For this review, take the finished solid that the model builds, in its own axes (mm). Coordinates: 2 decimals unless noted, no trailing zeros. Write each loop counter-clockwise with the first axis right and the second up, starting at its lowest first coordinate (ties: lowest second). Pieces come first, ordered by that corner, then holes. Notation, with made-up numbers: (79.25, 82.25) -> (118.25, 82.25) arc R12 cw to (118.25, 94.25) -> close; hole circle Ø3 at (29.5, 40.5). An arc over 180 degrees is marked (long way). Put each result on its own line as item: value. Start each with the question number.
Item 1: To check wall thickness, follow L1, parallel to X at y = -27, z = 11; L2, parallel to Z at x = 126, y = -24. State the ranges of each line that lie inside material, in increasing order.
Item 2: Consider section B-B on y = -17.5. Give the boundary of the cut face in (x, z).
Item 3: Insertion check: P1, Ø5, axis at y = -27.5, z = 28, coming from the +X side; P2, Ø5, axis at y = -51, z = 34.5, coming from the +X side; P3, Ø1, axis at y = -68, z = 18, coming from the +X side. Each pin has a flat end and moves straight along its axis. Give the tip position at first contact, or say it passes through.
Item 4: Consider section A-A on z = 40. Give the boundary of the cut face in (x, y).
Item 5: The part is to be moulded in two halves that separate along Y. For faces 1 (the flat face through (62, 0, 22)), 2 (the cylindrical face through (130.739, -27.575, 22.656)), 3 (the cylindrical face through (133.556, -60.157, 23.441)), 4 (the flat face through (138.43, -27, 27)), say which applies: +Y half, -Y half, draft (parallel to the pull), parting line (faces both ways), or undercut.
```python
from build123d import *

# Parameters (mm, degrees)
F0_W     = 125.73
F0_H     = 43.18
F1_DEPTH = 80.518
F2_R     = 6.35
F3_DEPTH = 19.05
F2_R_2   = 4.7625
F4_DEPTH = 12.7
F5_R     = 3.175
F6_R     = 2.54


with BuildPart() as f1:
    # F0 (on Front) → F1 (new body)
    with BuildSketch(Plane.XZ):
        with Locations((62.865, 21.59)):
            Rectangle(F0_W, F0_H)
    extrude(amount=F1_DEPTH)

    # F2 (on face) → F3 (join)
    with BuildSketch(Plane.YZ.offset(125.73)):
        with Locations((-55.118, 27.305)):
            Circle(F2_R)
    extrude(amount=F3_DEPTH)

    # F2 (on face) → F4 (join)
    with BuildSketch(Plane.YZ.offset(125.73)):
        with Locations((-26.543, 27.305)):
            Circle(F2_R_2)
    extrude(amount=F4_DEPTH)

    # F5
    f5_edges = [f1.edges().sort_by_distance(p)[0] for p in [
        (144.78, -61.468, 27.305),
    ]]
    fillet(f5_edges, radius=F5_R)

    # F6
    f6_edges = [f1.edges().sort_by_distance(p)[0] for p in [
        (138.43, -31.3055, 27.305),
    ]]
    fillet(f6_edges, radius=F6_R)


solid = f1.part
```
Return value:
1. L1: 0 to 125.73
1. L2: 23.28 to 31.33
2. outline: (0, 0) -> (125.73, 0) -> (125.73, 43.18) -> (0, 43.18) -> close
3. P1: x = 138.43
3. P2: x = 143.41
3. P3: x = 125.73
4. outline: (0, -80.52) -> (125.73, -80.52) -> (125.73, 0) -> (0, 0) -> close
5. face 1: +Y half
5. face 2: undercut
5. face 3: undercut
5. face 4: draft
